from build123d import *

# Parameters (mm, degrees)
EXTRUDE_1_DEPTH     = 30
SKETCH_2_W          = 10
SKETCH_2_H          = 4
CUT_EXTRUDE_1_DEPTH = 46
CHAMFER_1_SIZE      = 2
CHAMFER_2_SIZE      = 2
CHAMFER_3_SIZE      = 2


with BuildPart() as part:
    # 草图1 → 凸台-拉伸1 (new body)
    with BuildSketch(Plane.XY):
        with BuildLine():
            Line((8.5, 15), (15, 15))
            Line((15, 15), (15, -15))
            Line((15, -15), (-15, -15))
            Line((-15, -15), (-15, 15))
            Line((-15, 15), (-8.5, 15))
            ThreePointArc((-8.5, 15), (0, 6.5), (8.5, 15))
        make_face()
    extrude(amount=EXTRUDE_1_DEPTH)

    # 草图2 → 切除-拉伸1 (cut, through all)
    with BuildSketch(Plane(origin=(15, 0, 0), x_dir=(0, 0, -1), z_dir=(1, 0, 0))):
        with Locations((-15, 0)):
            Rectangle(SKETCH_2_W, SKETCH_2_H)
    extrude(amount=-CUT_EXTRUDE_1_DEPTH, mode=Mode.SUBTRACT)

    # 倒角1
    chamfer_1_edges = [part.edges().sort_by_distance(p)[0] for p in [
        (-15, 15, 15),
        (15, 15, 15),
    ]]
    chamfer(chamfer_1_edges, length=CHAMFER_1_SIZE)

    # 倒角2
    chamfer_2_edges = [part.edges().sort_by_distance(p)[0] for p in [
        (15, -15, 15),
        (-15, -15, 15),
    ]]
    chamfer(chamfer_2_edges, length=CHAMFER_2_SIZE)

    # 倒角3
    chamfer_3_edges = [part.edges().sort_by_distance(p)[0] for p in [
        (-15, 0, 0),
        (-15, 0, 30),
        (15, 0, 30),
        (15, 0, 0),
    ]]
    chamfer(chamfer_3_edges, length=CHAMFER_3_SIZE)


solid = part.part
CAD build for the part. Positions are in the model's coordinates, mm. A direction names the side the tool comes from. Coordinates: 2 decimals unless noted, no trailing zeros. Order: outer loops, then holes, each group sorted by start corner. A loop starts at its lowest first (then second) coordinate and runs counter-clockwise, first axis right, second up. Notation, with made-up numbers: (77, 56.25) -> (96, 56.25) arc R26 cw to (96, 90.25) -> close; hole circle Ø1 at (-20.5, -22). An arc over 180 degrees is marked (long way). Answer in a Markdown table with one row per item.
1) Mould opens along Y. For faces 1 (the face through (0, 0, 10)), 2 (the face through (14, 0, 1)), 3 (the face through (0, -15, 15)) say: pulls with the +Y half, pulls with the -Y half, needs draft (parallel to the pull), parting line crosses it, or undercut.
Check values:
| item | result |
|---|---|
| face 1 | undercut |
| face 2 | needs draft |
| face 3 | pulls with the -Y half |
2) Which spindle directions (+Z, -Z, +X, -X, +Y, -Y) get a long thin tool onto all of the face, cutting with end or side? Do faces 4 (the face through (0, -3, 0)), 5 (the face through (0, 2, 15)). Say none if no direction does.
Check values:
| item | result |
|---|---|
| face 4 | -Z, +X, -X, +Y, -Y |
| face 5 | +X, -X |
3) Band-saw the part on D-D (z = 22). List the corners of the cut face in (x, y), and give its area (3 significant figures).
Check values:
| item | result |
|---|---|
| outline | (-15, -13) -> (-13, -15) -> (13, -15) -> (15, -13) -> (15, 13) -> (13, 15) -> (8.5, 15) arc R8.5 cw to (-8.5, 15) -> (-13, 15) -> (-15, 13) -> close |
| area | 779 mm2 |
4) Band-saw the part on B-B (y = -0.75). List the corners of the cut face in (x, z).
Check values:
| item | result |
|---|---|
| outline | (-15, 2) -> (-13, 0) -> (13, 0) -> (15, 2) -> (15, 10) -> (-15, 10) -> close; (-15, 20) -> (15, 20) -> (15, 28) -> (13, 30) -> (-13, 30) -> (-15, 28) -> close |
5) Flat gauge pin, fed straight in: P1, Ø8, axis at x = -0.5, z = 13, coming from the +Y side. Where does the tip first touch, or does it go through?
Check values:
| item | result |
|---|---|
| P1 | y = 7.79 |
6) Band-saw the part on C-C (x = 0). List the corners of the cut face in (y, z).
Check values:
| item | result |
|---|---|
| outline | (-15, 0) -> (6.5, 0) -> (6.5, 30) -> (-15, 30) -> close; hole (-2, 10) -> (2, 10) -> (2, 20) -> (-2, 20) -> close |
7) Drill centre lines: line 1 (Y direction, x = -10.5, z = 16.25); line 2 (Y direction, x = 3.25, z = 11.75); line 3 (Z direction, x = -5.5, y = -1.5). Where is each one in solid material? Low to high.
Check values:
| item | result |
|---|---|
| line 1 | -15 to -2, 2 to 15 |
| line 2 | -15 to -2, 2 to 7.15 |
| line 3 | 0 to 10, 20 to 30 |
8) Band-saw the part on A-A (z = 12). List the corners of the cut face in (x, y).
Check values:
| item | result |
|---|---|
| outline | (-15, -13) -> (-13, -15) -> (13, -15) -> (15, -13) -> (15, -2) -> (-15, -2) -> close; (-15, 2) -> (15, 2) -> (15, 13) -> (13, 15) -> (8.5, 15) arc R8.5 cw to (-8.5, 15) -> (-13, 15) -> (-15, 13) -> close |
